```python
from build123d import *

# Parameters (mm, degrees)
SKETCH25_W          = 7
SKETCH25_H          = 8
BOSS_EXTRUDE5_DEPTH = 12.8
SKETCH26_W          = 24
SKETCH26_H          = 8
SKETCH26_R          = 2.65
BOSS_EXTRUDE6_DEPTH = 12
SKETCH27_R          = 1.55
CUT_EXTRUDE1_DEPTH  = 6.5
SKETCH29_R          = 1.625
BOSS_EXTRUDE8_DEPTH = 2.5
SKETCH31_W          = 24
SKETCH31_H          = 8
BOSS_EXTRUDE9_DEPTH = 1.5
FILLET1_R           = 2


with BuildPart() as part:
    # Sketch25 → Boss-Extrude5 (new body)
    with BuildSketch(Plane(origin=(0, 0, 0), x_dir=(-1, 0, 0), z_dir=(0, 1, 0))):
        Rectangle(SKETCH25_W, SKETCH25_H)
    extrude(amount=BOSS_EXTRUDE5_DEPTH)

    # Sketch26 → Boss-Extrude6 (add)
    with BuildSketch(Plane(origin=(0, 0, 0), x_dir=(-1, 0, 0), z_dir=(0, 1, 0))):
        Rectangle(SKETCH26_W, SKETCH26_H)
        with Locations(Location((-8, 0, 0), (0, 0, 90))):
            Circle(SKETCH26_R, mode=Mode.SUBTRACT)
        with Locations(Location((8, 0, 0), (0, 0, 90))):
            Circle(SKETCH26_R, mode=Mode.SUBTRACT)
    extrude(amount=BOSS_EXTRUDE6_DEPTH)

    # Sketch27 → Cut-Extrude1 (cut)
    with BuildSketch(Plane(origin=(0, 12.8, 0), x_dir=(1, 0, 0), z_dir=(0, 1, 0))):
        with Locations(Location((0, 0, 0), (0, 0, 270))):
            Circle(SKETCH27_R)
    extrude(amount=-CUT_EXTRUDE1_DEPTH, mode=Mode.SUBTRACT)

    # Sketch29 → Boss-Extrude8 (add)
    # profile 1 of 2: a face of its own
    with BuildSketch(Plane.XZ):
        with BuildLine():
            Line((-16.813742475, -2.303179977), (-12, 0.934295686))
            Line((-12, 0.934295686), (-12, -4))
            Line((-12, -4), (-7.689524447, -4))
            Line((-7.689524447, -4), (-13.186257525, -7.696820023))
            ThreePointArc((-13.186257525, -7.696820023), (-17.696820023, -6.813742475), (-16.813742475, -2.303179977))
        make_face()
        with Locations(Location((-15, -5, 0), (0, 0, 270))):
            Circle(SKETCH29_R, mode=Mode.SUBTRACT)
    # profile 2 of 2: a face of its own
    with BuildSketch(Plane.XZ):
        with BuildLine():
            Line((16.813742475, -2.303179977), (12, 0.934295686))
            Line((12, 0.934295686), (12, -4))
            Line((12, -4), (7.689524447, -4))
            Line((7.689524447, -4), (13.186257525, -7.696820023))
            ThreePointArc((13.186257525, -7.696820023), (17.696820023, -6.813742475), (16.813742475, -2.303179977))
        make_face()
        with Locations(Location((15, -5, 0), (0, 0, 90))):
            Circle(SKETCH29_R, mode=Mode.SUBTRACT)
    extrude(amount=-BOSS_EXTRUDE8_DEPTH)

    # Sketch31 → Boss-Extrude9 (add)
    with BuildSketch(Plane.XZ):
        Rectangle(SKETCH31_W, SKETCH31_H)
    extrude(amount=BOSS_EXTRUDE9_DEPTH)

    # Fillet1
    fillet1_edges = [part.edges().sort_by_distance(p)[0] for p in [
        (12, 7.25, -4),
        (-12, 5.25, 4),
        (12, 5.25, 4),
        (-12, 7.25, -4),
        (-12, -0.75, -4),
        (12, -0.75, -4),
    ]]
    fillet(fillet1_edges, radius=FILLET1_R)


solid = part.part
```
Part model, mm, in its own coordinate system. A direction names the side the tool comes from. Give positions to 0.01 mm unless a question says otherwise; leave off trailing zeros. Order: outer loops, then holes, each group sorted by start corner. A loop starts at its lowest first (then second) coordinate and runs counter-clockwise, first axis right, second up. Notation, with made-up numbers: M 4,67.5 L 22,67.5 A9 cw 22,71.5 Z; hole C 38,-37 d9. An arc over 180 degrees is marked long. Use a Markdown table: item, result. Add a question column.
(1) Saw through at A-A, the plane y = 7. Give the cut face in (x, z), and give its area (3 significant figures).
(2) 3-axis set-ups, long thin cutter, end or side, ignore diameter. For faces 1 (the face through (-3.5, 12.4, -0.1)), 2 (the face through (-10.59, 5.92, -0.57)), 3 (the face through (-11.43, -0.76, -3.4)): which of +Z, -Z, +X, -X, +Y, -Y reach the whole face in a straight line?
(3) Drop flat-ended pins along their axis: P1, Ø6, axis at x = -7.5, z = 0.5, coming from the +Y side; P2, Ø1, axis at y = 1, z = -6.5, coming from the -X side; P3, Ø4, axis at y = 10, z = -4, coming from the -X side; P4, Ø1, axis at x = 14.5, z = -4.5, coming from the +Y side. Give the stop position or say it passes through.
(4) Saw through at D-D, the plane z = 0. Give the cut face in (x, y), and give its area (3 significant figures).
(5) Probe line 1 along X through (y, z) = (8.25, 0); line 2 along X through (y, z) = (5, 0); line 3 along X through (y, z) = (11.5, 2.25). List the from-to ranges inside material, lowest first. Write a range as [from, to].
(6) Mould opens along X. For faces 4 (the face through (-10.399, 1.232, -5.823)), 5 (the face through (12, 7, 0)), 6 (the face through (-6, 12, 2)) say: +X half, -X half, draft (parallel to the pull), parting line (faces both ways), or undercut.
(7) Saw through at C-C, the plane z = -5. Give the cut face in (x, y) (3 decimals).
(8) Saw through at B-B, the plane x = 0. Give the cut face in (y, z), and give its area (4 significant figures).
Answer key:
| question | item | result |
|---|---|---|
| 1 | outline | M -12,-2 A2 ccw -10,-4 L 10,-4 A2 ccw 12,-2 L 12,2 A2 ccw 10,4 L -10,4 A2 ccw -12,2 Z; hole C -8,0 d5.3; hole C 0,0 d3.1; hole C 8,0 d5.3 |
| 1 | area | 137 mm^2 |
| 2 | face 1 | +Z, -Z, -X, +Y |
| 2 | face 2 | +Y |
| 2 | face 3 | -Z, -X, -Y |
| 3 | P1 | y = 12 |
| 3 | P2 | x = -18.09 |
| 3 | P3 | x = -12 |
| 3 | P4 | through |
| 4 | outline | M -13.39,0 L -12,0 L -12,-1.5 L 12,-1.5 L 12,0 L 13.39,0 L 13.39,2.5 L 12,2.5 L 12,12 L 10.65,12 L 10.65,0 L 5.35,0 L 5.35,12 L 3.5,12 L 3.5,12.8 L 1.55,12.8 L 1.55,6.3 L -1.55,6.3 L -1.55,12.8 L -3.5,12.8 L -3.5,12 L -5.35,12 L -5.35,0 L -10.65,0 L -10.65,12 L -12,12 L -12,2.5 L -13.39,2.5 Z |
| 4 | area | 189 mm^2 |
| 5 | line 1 | [-12, -10.65], [-5.35, -1.55], [1.55, 5.35], [10.65, 12] |
| 5 | line 2 | [-12, -10.65], [-5.35, 5.35], [10.65, 12] |
| 5 | line 3 | [-11.98, -9.4], [-6.6, 6.6], [9.4, 11.98] |
| 6 | face 4 | undercut |
| 6 | face 5 | +X half |
| 6 | face 6 | draft |
| 7 | outline | M -18.25,0 L -16.625,0 L -16.625,2.5 L -18.25,2.5 Z; M -13.375,0 L -9.176,0 L -9.176,2.5 L -13.375,2.5 Z; M 9.176,0 L 13.375,0 L 13.375,2.5 L 9.176,2.5 Z; M 16.625,0 L 18.25,0 L 18.25,2.5 L 16.625,2.5 Z |
| 8 | outline | M -1.5,-4 L 12.8,-4 L 12.8,-1.55 L 6.3,-1.55 L 6.3,1.55 L 12.8,1.55 L 12.8,4 L -1.5,4 Z |
| 8 | area | 94.25 mm^2 |
